```python
from build123d import *

# Parameters (mm, degrees)
F0_W     = 70
F0_H     = 44.7
F1_DEPTH = 21.77
F2_R     = 2.5527
F3_DEPTH = 15
F4_W     = 2
F4_H     = 44.7
F5_DEPTH = 2


with BuildPart() as f1:
    # F0 (on Top) → F1 (new body)
    with BuildSketch(Plane.XY):
        with Locations((35, 22.35)):
            Rectangle(F0_W, F0_H)
    extrude(amount=F1_DEPTH)

    # F2 (on face) → F3 (cut)
    with BuildSketch(Plane.XY.offset(21.77)):
        with Locations((40.014, 22.587)):
            Circle(F2_R)
    extrude(amount=-F3_DEPTH, mode=Mode.SUBTRACT)

    # F4 (on face) → F5 (cut)
    with BuildSketch(Plane(origin=(0, 0, 0), x_dir=(1, 0, 0), z_dir=(0, 0, -1))):
        with Locations((67, -22.35)):
            Rectangle(F4_W, F4_H)
        with Locations((60.75, -22.35)):
            Rectangle(F4_W, F4_H)
        with Locations((54.5, -22.35)):
            Rectangle(F4_W, F4_H)
        with Locations((48.25, -22.35)):
            Rectangle(F4_W, F4_H)
        with Locations((42, -22.35)):
            Rectangle(F4_W, F4_H)
        with Locations((35.75, -22.35)):
            Rectangle(F4_W, F4_H)
        with Locations((29.5, -22.35)):
            Rectangle(F4_W, F4_H)
        with Locations((23.25, -22.35)):
            Rectangle(F4_W, F4_H)
        with Locations((17, -22.35)):
            Rectangle(F4_W, F4_H)
        with Locations((10.75, -22.35)):
            Rectangle(F4_W, F4_H)
        with Locations((4.5, -22.35)):
            Rectangle(F4_W, F4_H)
        with Locations((-1.75, -22.35)):
            Rectangle(F4_W, F4_H)
    extrude(amount=-F5_DEPTH, mode=Mode.SUBTRACT)


solid = f1.part
```
Can you work these out from the model? Positions are in its coordinate system, mm. A direction names the side the tool comes from. Round coordinates to 2 decimals unless told otherwise and drop trailing zeros. Order: outer loops, then holes, each group sorted by start corner. A loop starts at its lowest first (then second) coordinate and runs counter-clockwise, first axis right, second up. Notation, with made-up numbers: (53, -9.5) -> (83, -9.5) arc R19 cw to (83, -3.5) -> close; hole circle Ø6 at (-12, 58). An arc over 180 degrees is marked (long way). Return JSON: item names as keys, results as strings. Group by question number.
1. We'd pull the mould along Y, two halves only. Please class faces 3 (the face through (40, 23, 6.77)), 4 (the face through (20, 23, 0)): released by +Y, released by -Y, zero draft, split by the parting line, or undercut.
2. If we section it at A-A, the plane x = 29.5: Write out the boundary of the cut face in (y, z), then the cut area to 3 significant figures.
3. Will this pin go through, and if not, where does the flat tip stop? pin 1 (1 mm diameter, centred on x = 60.5, y = 28.5, fed in from -Z).
4. I need wall thicknesses on line 1 (X direction, y = 20.5, z = 17.75); line 2 (Z direction, x = 61.5, y = 34.5). Which ranges of each line are inside material? Lowest first, please. Write a range as [from, to].
5. Which directions (+Z, -Z, +X, -X, +Y, -Y) give clear straight access to the entire face, cutting with the end or side of a thin tool? Please do faces 1 (the face through (3.5, 23, 1)), 2 (the face through (58, 23, 0)).
Output values:
{
 "1": {"face 3": "undercut", "face 4": "zero draft"},
 "2": {"outline": "(0, 2) -> (44.7, 2) -> (44.7, 21.77) -> (0, 21.77) -> close", "area": "884 mm²"},
 "3": {"pin 1": "z = 2"},
 "4": {"line 1": "[0, 38.54], [41.48, 70]", "line 2": "[2, 21.77]"},
 "5": {"face 1": "-Z, +Y, -Y", "face 2": "-Z, +X, -X, +Y, -Y"}
}
